```python
from build123d import *

# Parameters (mm, degrees)
SKETCH1_W          = 100
SKETCH1_H          = 60
BASE_FLANGE1_DEPTH = 1.89738
SKETCH7_R          = 2
CUT_EXTRUDE2_DEPTH = 2


# Sheet-metal steps are written as plain solids
with BuildPart() as part:
    # Sketch1 → Base-Flange1 (new body)
    with BuildSketch(Plane.XY):
        with Locations((-16.008698092, 3.086666862)):
            Rectangle(SKETCH1_W, SKETCH1_H)
    extrude(amount=-BASE_FLANGE1_DEPTH)

    # Sketch7 → Cut-Extrude2 (cut)
    with BuildSketch(Plane.XY):
        with Locations((-16.008698092, 3.086666862)):
            Circle(SKETCH7_R)
        with BuildLine():
            Line((-60.644357263, -9.061184979), (-55.644357263, -9.061184979))
            ThreePointArc((-55.644357263, -9.061184979), (-53.144357263, -11.561184979), (-55.644357263, -14.061184979))
            Line((-55.644357263, -14.061184979), (-60.644357263, -14.061184979))
            ThreePointArc((-60.644357263, -14.061184979), (-63.144357263, -11.561184979), (-60.644357263, -9.061184979))
        make_face()
        with BuildLine():
            Line((-60.644357263, 25.938815021), (-55.644357263, 25.938815021))
            ThreePointArc((-55.644357263, 25.938815021), (-53.144357263, 23.438815021), (-55.644357263, 20.938815021))
            Line((-55.644357263, 20.938815021), (-60.644357263, 20.938815021))
            ThreePointArc((-60.644357263, 20.938815021), (-63.144357263, 23.438815021), (-60.644357263, 25.938815021))
        make_face()
        with BuildLine():
            Line((27.560882737, 20.938815021), (22.560882737, 20.938815021))
            ThreePointArc((22.560882737, 20.938815021), (20.060882737, 23.438815021), (22.560882737, 25.938815021))
            Line((22.560882737, 25.938815021), (27.560882737, 25.938815021))
            ThreePointArc((27.560882737, 25.938815021), (30.060882737, 23.438815021), (27.560882737, 20.938815021))
        make_face()
        with BuildLine():
            Line((27.560882737, -14.061184979), (22.560882737, -14.061184979))
            ThreePointArc((22.560882737, -14.061184979), (20.060882737, -11.561184979), (22.560882737, -9.061184979))
            Line((22.560882737, -9.061184979), (27.560882737, -9.061184979))
            ThreePointArc((27.560882737, -9.061184979), (30.060882737, -11.561184979), (27.560882737, -14.061184979))
        make_face()
    extrude(amount=-CUT_EXTRUDE2_DEPTH, mode=Mode.SUBTRACT)


solid = part.part
```
Design review of the part built by this model. Coordinates are the model's own, in mm. A direction names the side the tool comes from. Give positions to 0.01 mm unless a question says otherwise; leave off trailing zeros. Loops run counter-clockwise (first coordinate to the right, second up) from the corner with the lowest first, then second, coordinate; pieces in that order, holes last. Notation, with made-up numbers: (66, 70.25) -> (76, 70.25) arc R8 cw to (76, 75.25) -> close; hole circle Ø11 at (78, -29.5). An arc over 180 degrees is marked (long way). Write each question's results on one line, items separated by ' | '.
Q1. Take a section at B-B, the plane z = -0.6. Write out the cut boundary in (x, y).
Reply:
outline: (-66.01, -26.91) -> (33.99, -26.91) -> (33.99, 33.09) -> (-66.01, 33.09) -> close; hole (-60.64, -14.06) -> (-55.64, -14.06) arc R2.5 ccw to (-55.64, -9.06) -> (-60.64, -9.06) arc R2.5 ccw to start; hole (-60.64, 20.94) -> (-55.64, 20.94) arc R2.5 ccw to (-55.64, 25.94) -> (-60.64, 25.94) arc R2.5 ccw to start; hole circle Ø4 at (-16.01, 3.09); hole (22.56, -14.06) -> (27.56, -14.06) arc R2.5 ccw to (27.56, -9.06) -> (22.56, -9.06) arc R2.5 ccw to start; hole (22.56, 20.94) -> (27.56, 20.94) arc R2.5 ccw to (27.56, 25.94) -> (22.56, 25.94) arc R2.5 ccw to start
Q2. The part is to be moulded in two halves that separate along X. For faces 1 (the face through (30.06, -11.51, -0.94)), 2 (the face through (-53.145, 23.494, -0.935)), 3 (the face through (33.991, 3, -1)), 4 (the face through (-17, -3, -1.897)), say which applies: +X half, -X half, draft (parallel to the pull), parting line (faces both ways), or undercut.
Reply:
face 1: undercut | face 2: undercut | face 3: +X half | face 4: draft
Q3. Take a section at A-A, the plane y = -12.5. Write out the cut boundary in (x, z), plus the area to 3 significant figures.
Reply:
outline: (-66.01, -1.9) -> (-62.96, -1.9) -> (-62.96, 0) -> (-66.01, 0) -> close; (-53.33, -1.9) -> (20.24, -1.9) -> (20.24, 0) -> (-53.33, 0) -> close; (29.88, -1.9) -> (33.99, -1.9) -> (33.99, 0) -> (29.88, 0) -> close | area: 153 mm²
Q4. Take a section at C-C, the plane y = 24.5. Write out the cut boundary in (x, z).
Reply:
outline: (-66.01, -1.9) -> (-62.91, -1.9) -> (-62.91, 0) -> (-66.01, 0) -> close; (-53.38, -1.9) -> (20.3, -1.9) -> (20.3, 0) -> (-53.38, 0) -> close; (29.82, -1.9) -> (33.99, -1.9) -> (33.99, 0) -> (29.82, 0) -> close
Q5. Wall thickness on L1, parallel to Y at x = -56, z = -1.15; L2, parallel to X at y = 3, z = -0.65; L3, parallel to X at y = 24.5, z = -1: over which ranges is each line inside the solid? List them lowest first.
Reply:
L1: y = -26.91 to -14.06, -9.06 to 20.94, 25.94 to 33.09 | L2: x = -66.01 to -18.01, -14.01 to 33.99 | L3: x = -66.01 to -62.91, -53.38 to 20.3, 29.82 to 33.99
Q6. Machinability: for faces 5 (the face through (-66.009, 3, -1)), 6 (the face through (-58, 20.939, -1)), which of the approach directions +Z, -Z, +X, -X, +Y, -Y give a long, thin tool a straight path to every point of the face, cutting with its end or side? Answer none if there is none.
Reply:
face 5: +Z, -Z, -X, +Y, -Y | face 6: +Z, -Z
